For this review, use the dimensioned drawing (mm, ordinates from the lowest corner) and the shaded views. Give positions to 0.01 mm unless a question says otherwise; leave off trailing zeros. Write each loop counter-clockwise with the first axis right and the second up, starting at its lowest first coordinate (ties: lowest second). Pieces come first, ordered by that corner, then holes. Notation, with made-up numbers: (39, 51.25) -> (96, 51.25) arc R20 ccw to (96, 86.25) -> close; hole circle Ø3 at (82, 77). An arc over 180 degrees is marked (long way). Return JSON: item names as keys, results as strings.
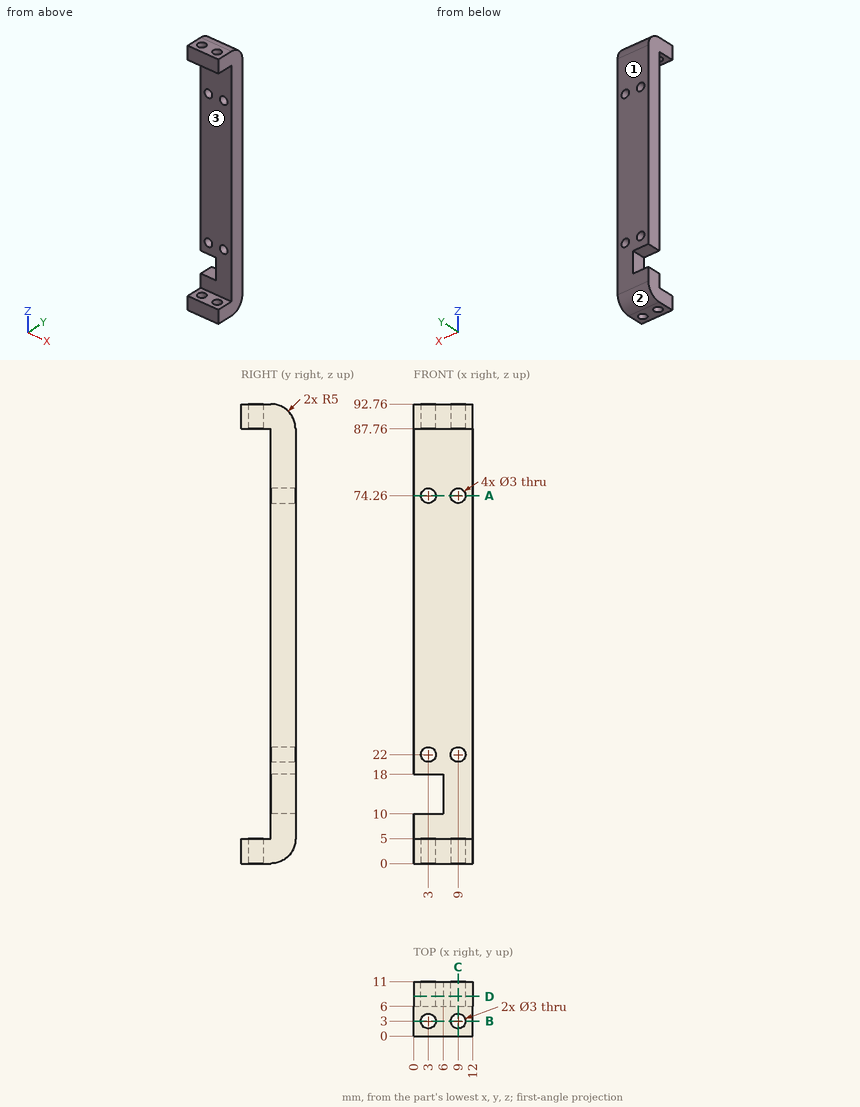
1. The part is to be moulded in two halves that separate along Z. For the marked faces 1, 2 and 3, say which applies: +Z half, -Z half, draft (parallel to the pull), parting line (faces both ways), or undercut.
Results found:
{"face 1": "draft", "face 2": "-Z half", "face 3": "undercut"}
2. For pin 1 (5 mm diameter, centred on x = 9, y = 3, fed in from +Z); pin 2 (3.5 mm diameter, centred on x = 3, z = 74.26, fed in from -Y); pin 3 (2.5 mm diameter, centred on x = 3.5, y = 8, fed in from +Z); pin 4 (4 mm diameter, centred on y = 8, z = 13.5, fed in from -X), all flat-tipped, find the tip position at first contact; note any pin that passes through.
Results found:
{"pin 1": "stops at z = 92.76", "pin 2": "stops at y = 6", "pin 3": "stops at z = 92.7", "pin 4": "stops at x = 6"}
3. To check wall thickness, follow probe 1 along X at (y, z) = (9.95, 22); probe 2 along Z at (x, y) = (4.75, 3); probe 3 along Y at (x, z) = (7, 17). State the ranges of each line that lie inside material, in increasing order.
Results found:
{"probe 1": "x = 0 to 1.5, 4.5 to 7.5, 10.5 to 12", "probe 2": "z = 0 to 5, 87.76 to 92.76", "probe 3": "y = 6 to 11"}
4. Add section A-A, the plane z = 74.26. State the section outline as (x, y) points, plus the area to 3 significant figures.
Results found:
{"outline": "(0, 6) -> (1.5, 6) -> (1.5, 11) -> (0, 11) -> close; (4.5, 6) -> (7.5, 6) -> (7.5, 11) -> (4.5, 11) -> close; (10.5, 6) -> (12, 6) -> (12, 11) -> (10.5, 11) -> close", "area": "30.0 mm²"}
5. Add section D-D, the plane y = 8. State the section outline as (x, z) points.
Results found:
{"outline": "(0, 0.42) -> (12, 0.42) -> (12, 92.34) -> (0, 92.34) -> (0, 18) -> (6, 18) -> (6, 10) -> (0, 10) -> close; hole circle Ø3 at (3, 22); hole circle Ø3 at (3, 74.26); hole circle Ø3 at (9, 22); hole circle Ø3 at (9, 74.26)"}
6. Add section C-C, the plane x = 9. State the section outline as (y, z) points.
Results found:
{"outline": "(0, 0) -> (1.5, 0) -> (1.5, 5) -> (0, 5) -> close; (0, 87.76) -> (1.5, 87.76) -> (1.5, 92.76) -> (0, 92.76) -> close; (4.5, 0) -> (6, 0) arc R5 ccw to (11, 5) -> (11, 20.5) -> (6, 20.5) -> (6, 5) -> (4.5, 5) -> close; (4.5, 87.76) -> (6, 87.76) -> (6, 75.76) -> (11, 75.76) -> (11, 87.76) arc R5 ccw to (6, 92.76) -> (4.5, 92.76) -> close; (6, 23.5) -> (11, 23.5) -> (11, 72.76) -> (6, 72.76) -> close"}
7. Add section B-B, the plane y = 3. State the section outline as (x, z) points.
Results found:
{"outline": "(0, 0) -> (1.5, 0) -> (1.5, 5) -> (0, 5) -> close; (0, 87.76) -> (1.5, 87.76) -> (1.5, 92.76) -> (0, 92.76) -> close; (4.5, 0) -> (7.5, 0) -> (7.5, 5) -> (4.5, 5) -> close; (4.5, 87.76) -> (7.5, 87.76) -> (7.5, 92.76) -> (4.5, 92.76) -> close; (10.5, 0) -> (12, 0) -> (12, 5) -> (10.5, 5) -> close; (10.5, 87.76) -> (12, 87.76) -> (12, 92.76) -> (10.5, 92.76) -> close"}
